Autodesk Inventor part; units mm, degrees
ref_plane "YZ Plane" through (0, 0, 0) normal (1, 0, 0) x (0, 1, 0)
ref_plane "XZ Plane" through (0, 0, 0) normal (0, 1, 0) x (-1, 0, 0)
ref_plane "XY Plane" through (0, 0, 0) normal (0, 0, 1) x (1, 0, 0)
sketch "Sketch2" plane through (0, 0, 0) normal (0, 0, 1) x (1, 0, 0)
  circle A0 centre (0, 0) radius 4
  line L0 (-4, 0) -> (4, 0)
  line L1 (4, 0) -> (4, 25)
  line L2 (4, 25) -> (-4, 25)
  line L3 (-4, 25) -> (-4, 0)
  point P0 (4, 0)
  dimension "d11" = 8
  dimension "d12" = 8
  dimension "d13" = 25
extrude "Extrusion2" add sketch "Sketch2" along normal blind 5
sketch "Sketch3" plane through (0, 0, 5) normal (0, 0, 1) x (1, 0, 0)
  line L0 (4, 0) -> (4, 25)
  line L1 (-16, 27.5) -> (4, 27.5)
  line L2 (4, 27.5) -> (4, 22.5)
  line L3 (4, 22.5) -> (-16, 22.5)
  line L4 (-16, 22.5) -> (-16, 27.5)
  line L5 (4, 25) -> (-4, 25)
  point P0 (0, 0)
  point P1 (3, 25)
  dimension "d16" = 2.5
  dimension "d17" = 2.5
  dimension "d18" = 20
extrude "Extrusion3" add sketch "Sketch3" against normal blind 5
sketch "Sketch4" plane through (0, 0, 5) normal (0, 0, 1) x (1, 0, 0)
  line L0 (4, 0) -> (4, 27.5)
  line L1 (-16, 22.5) -> (-16, 27.5)
  line L2 (4, 27.5) -> (-16, 27.5)
  line L3 (-16, 27.5) -> (-16, 22.5)
  line L4 (-16, 22.5) -> (4, 22.5)
  line L5 (4, 22.5) -> (4, 27.5)
  point P0 (0, 0)
extrude "Extrusion4" add sketch "Sketch4" along normal blind 3
sketch "Sketch6" plane through (0, 0, 0) normal (0, 0, -1) x (-1, 0, 0)
  circle A0 centre (0, 0) radius 3.5
  dimension "d30" = 7
extrude "Extrusion6" cut sketch "Sketch6" against normal blind 5
sketch "Sketch7" plane through (0, 0, 0) normal (0, 0, -1) x (-1, 0, 0)
  line L0 (-3.2, -6) -> (3.2, -6)
  line L1 (3.2, -6) -> (3.2, -1)
  line L2 (3.2, -1) -> (-3.2, -1)
  line L3 (-3.2, -1) -> (-3.2, -6)
  line L4 (-4, 0) -> (-4, 27.5)
  line L5 (4, 22.5) -> (4, 0)
  point P0 (0, 0)
  point P1 (-4, 24.5)
  dimension "d33" = 1
  dimension "d34" = 6
  dimension "d35" = 0.8
  dimension "d36" = 0.8
extrude "Extrusion7" cut sketch "Sketch7" against normal blind 5
sketch "Sketch8" plane through (0, 0, 0) normal (0, 0, -1) x (-1, 0, 0)
  circle A0 centre (0, 16) radius 2.1
  arc A1 (3.2, -1.4177) -> (-3.2, -1.4177) centre (0, 0) ccw
  line L0 (-3.5, 0) -> (-2.1, 16)
  line L1 (2.1, 16) -> (3.4864, 0.308)
  point P0 (-3.4468, 0.6078)
  dimension "d39" = 16
  dimension "d40" = 4.2
extrude "Extrusion8" cut sketch "Sketch8" against normal blind 5 contours A0 | L1 A1 L0 A0
sketch "Sketch10" plane through (0, 0, 5) normal (0, 0, 1) x (1, 0, 0)
  line L0 (-4, 22.5) -> (-4, 0)
  line L1 (4, 0) -> (4, 22.5)
  line L2 (-4, 22.5) -> (4, 22.5)
  line L3 (4, 22.5) -> (4, 0)
  line L4 (4, 0) -> (-4, 0)
  line L5 (-4, 0) -> (-4, 22.5)
  point P0 (0, 0)
  point P1 (-4, 15.5)
  point P2 (-4, 15.5)
  point P3 (-4, 14.5)
extrude "Extrusion10" add sketch "Sketch10" along normal blind 3
chamfer "Chamfer5" distance 7 angle 45 1 edges at (-4, 22.5, 4)
chamfer "Chamfer6" distance 11 angle 45 1 edges at (4, 27.5, 4)
fillet "Fillet6" radius 5 2 edges at (-7, 27.5, 4) (4, 16.5, 4)
fillet "Fillet7" radius 2 2 edges at (-11, 22.5, 4) (-4, 15.5, 4)
sketch "Sketch14" plane through (0, 0, 5) normal (0, 0, 1) x (1, 0, 0)
  circle A0 centre (0, 0) radius 4
extrude "Extrusion14" add sketch "Sketch14" along normal blind 3
sketch "Sketch15" plane through (0, 0, 8) normal (0, 0, 1) x (1, 0, 0)
  line L0 (-16, 22.5) -> (-16, 27.5)
  line L1 (-16, 27.5) -> (-16, 22.5)
  line L2 (-16, 22.5) -> (-14.7, 22.5)
  line L3 (-11.8284, 22.5) -> (-16, 22.5)
  line L4 (-16, 27.5) -> (-14.7, 22.5)
  point P0 (0, 0)
  dimension "d82" = 1.3
extrude "Extrusion15" cut sketch "Sketch15" against normal blind 20
properties part number "switch-pusher"
Part model, mm, in its own coordinate system. A direction names the side the tool comes from. Coordinates: 2 decimals unless noted, no trailing zeros. Order: outer loops, then holes, each group sorted by start corner. A loop starts at its lowest first (then second) coordinate and runs counter-clockwise, first axis right, second up. Notation, with made-up numbers: M 55.5,-30.75 L 93.5,-30.75 A8 ccw 93.5,-20.75 Z; hole C -2,57.5 d6. An arc over 180 degrees is marked long. Use a Markdown table: item, result.
(1) Probe L1, parallel to Z at x = -0.5, y = 9; L2, parallel to Y at x = -13.5, z = 3; L3, parallel to X at y = 5, z = 6.75. List the from-to ranges inside material, lowest first.
A:
| item | result |
|---|---|
| L1 | z = 5 to 8 |
| L2 | y = 22.5 to 27.5 |
| L3 | x = -4 to 4 |
(2) Cut at C-C on y = 11. Write the cut outline in (x, z), then the cut area to 3 significant figures.
A:
| item | result |
|---|---|
| outline | M -4,0 L -2.54,0 L -2.54,5 L 2.54,5 L 2.54,0 L 4,0 L 4,8 L -4,8 Z |
| area | 38.6 mm^2 |
(3) Pull direction X, two halves, no side cores. Call faces 4 (the flat face through (-3.2, -2, 2)), 5 (the flat face through (-5, 19, 0)), 6 (the cylindrical face through (3.63, 16.32, 4.06)): released by +X, released by -X, zero draft, split by the parting line, or undercut.
A:
| item | result |
|---|---|
| face 4 | undercut |
| face 5 | zero draft |
| face 6 | released by +X |
(4) Cut at D-D on x = -5. Write the cut outline in (y, z).
A:
| item | result |
|---|---|
| outline | M 16.5,0 L 25.5,0 L 25.5,8 L 16.5,8 Z |
(5) Flat gauge pins, fed straight in: pin 1 (0.5 mm diameter, centred on y = -2, z = 2.5, fed in from +X); pin 2 (3 mm diameter, centred on y = 23, z = 1, fed in from -X); pin 3 (1 mm diameter, centred on y = 12.5, z = 6, fed in from -X). Where does each tip first touch, or does it go through?
A:
| item | result |
|---|---|
| pin 1 | stops at x = 3.6 |
| pin 2 | stops at x = -15.22 |
| pin 3 | stops at x = -4 |
(6) Cut at A-A on z = 5.5. Write the cut outline in (x, y), then the cut area to 3 significant figures.
A:
| item | result |
|---|---|
| outline | M -16,27.5 L -14.7,22.5 L -11.83,22.5 A2 cw -10.41,21.91 L -4.59,16.09 A2 cw -4,14.67 L -4,0 A4 ccw 4,0 L 4,14.43 A5 ccw 2.54,17.96 L -5.54,26.04 A5 ccw -9.07,27.5 Z |
| area | 265 mm^2 |
(7) Cut at B-B on x = 0. Write the cut outline in (y, z), then the cut area to 3 significant figures.
A:
| item | result |
|---|---|
| outline | M -4,5 L 18.1,5 L 18.1,0 L 20.5,0 L 20.5,8 L -4,8 Z |
| area | 85.5 mm^2 |
(8) Tool access for faces 1 (the cylindrical face through (0, 18.1, 2.5)), 2 (the cylindrical face through (-11.07, 22.35, 3.94)), 3 (the flat face through (-2.783, 8.264, 2.465)): list every direction of +Z, -Z, +X, -X, +Y, -Y with a clear straight run to the whole face (end or side of a thin tool).
A:
| item | result |
|---|---|
| face 1 | -Z, -Y |
| face 2 | +Z, -Z, -X, -Y |
| face 3 | -Z |
